```python
from build123d import *

# Parameters (mm, degrees)
CROQUIS1_W              = 56.2
CROQUIS1_H              = 31.2
SALIENTE_EXTRUIR1_DEPTH = 6
CROQUIS3_W              = 51.9
CROQUIS3_H              = 26.9
CORTAR_EXTRUIR1_DEPTH   = 3
CROQUIS5_W              = 56.2
CROQUIS5_H              = 18
SALIENTE_EXTRUIR2_DEPTH = 8
CROQUIS6_W              = 13.3
CROQUIS6_H              = 3.9
CORTAR_EXTRUIR2_DEPTH   = 64.385171768
CROQUIS7_W              = 13.1
CROQUIS7_H              = 8
CORTAR_EXTRUIR3_DEPTH   = 57.729533754
REDONDEO3_R             = 3


with BuildPart() as part:
    # Croquis1 → Saliente-Extruir1 (new body)
    with BuildSketch(Plane(origin=(0, 0, 0), x_dir=(1, 0, 0), z_dir=(0, 1, 0))):
        with Locations((25.1, 12.6)):
            Rectangle(CROQUIS1_W, CROQUIS1_H)
    extrude(amount=SALIENTE_EXTRUIR1_DEPTH)

    # Croquis3 → Cortar-Extruir1 (cut)
    with BuildSketch(Plane(origin=(0, 6, 0), x_dir=(1, 0, 0), z_dir=(0, 1, 0))):
        with Locations((25.1, 12.6)):
            Rectangle(CROQUIS3_W, CROQUIS3_H)
    extrude(amount=-CORTAR_EXTRUIR1_DEPTH, mode=Mode.SUBTRACT)

    # Croquis5 → Saliente-Extruir2 (add)
    with BuildSketch(Plane.XZ):
        with Locations((25.1, -6)):
            Rectangle(CROQUIS5_W, CROQUIS5_H)
    extrude(amount=SALIENTE_EXTRUIR2_DEPTH)

    # Croquis6 → Cortar-Extruir2 (cut, through all)
    with BuildSketch(Plane.ZY.offset(3)):
        with Locations((-8.35, -1.95)):
            Rectangle(CROQUIS6_W, CROQUIS6_H)
    extrude(amount=-CORTAR_EXTRUIR2_DEPTH, mode=Mode.SUBTRACT)

    # Croquis7 → Cortar-Extruir3 (cut, through all)
    with BuildSketch(Plane(origin=(0, 0, -15), x_dir=(-1, 0, 0), z_dir=(0, 0, -1))):
        with Locations((-46.65, -4)):
            Rectangle(CROQUIS7_W, CROQUIS7_H)
        with Locations((-3.55, -4)):
            Rectangle(CROQUIS7_W, CROQUIS7_H)
    extrude(amount=-CORTAR_EXTRUIR3_DEPTH, mode=Mode.SUBTRACT)

    # Redondeo3
    redondeo3_edges = [part.edges().sort_by_distance(p)[0] for p in [
        (-3, 3, -28.2),
        (53.2, 3, -28.2),
        (53.2, 3, 3),
        (-3, 3, 3),
    ]]
    fillet(redondeo3_edges, radius=REDONDEO3_R)


solid = part.part
```
Check sheet for the modelled part. Datum: model origin and axes. Units: mm. A direction names the side the tool comes from. Round coordinates to 2 decimals unless told otherwise and drop trailing zeros. Loops run counter-clockwise (first coordinate to the right, second up) from the corner with the lowest first, then second, coordinate; pieces in that order, holes last. Notation, with made-up numbers: M -19,-9.75 L 2,-9.75 A11 ccw 2,6.25 Z; hole C 10,2.25 d11. An arc over 180 degrees is marked long. Answer as a JSON object with one key per item and string values.
1. Scan lines: line 1 (X direction, y = 4.25, z = -13); line 2 (Z direction, x = 46, y = 4); line 3 (Y direction, x = 27, z = -17.5). Record each from-to range of solid material in increasing order.
Reply:
{"line 1": "x = -3 to -0.85, 51.05 to 53.2", "line 2": "z = -28.2 to -26.05, 0.85 to 3", "line 3": "y = 0 to 3"}
2. Access from +Z, -Z, +X, -X, +Y, -Y to the whole of each face (thin tool, end or side, straight path). Record for faces 5 (the flat face through (51.05, 5, -12)), 6 (the flat face through (25, -3.9, -8)), 7 (the flat face through (25, -6, -15)), 8 (the flat face through (10.1, -5, -4)), 9 (the flat face through (-3, 3, -13)).
Reply:
{"face 5": "+Y", "face 6": "-Z, +X, -X", "face 7": "-Z, +X, -X, -Y", "face 8": "+Z, -Z, -X, -Y", "face 9": "+Z, -Z, -X, +Y, -Y"}
3. Section check D-D (y = -7). Record the boundary of the cut face in (x, z).
Reply:
{"outline": "M 10.1,-15 L 40.1,-15 L 40.1,3 L 10.1,3 Z"}
4. Section check C-C (z = -17.5). Record the boundary of the cut face in (x, y).
Reply:
{"outline": "M -3,0 L 53.2,0 L 53.2,6 L 51.05,6 L 51.05,3 L -0.85,3 L -0.85,6 L -3,6 Z"}
5. Section check A-A (z = -11.5). Record the boundary of the cut face in (x, y), plus the area to 4 significant figures.
Reply:
{"outline": "M -3,0 L 53.2,0 L 53.2,6 L 51.05,6 L 51.05,3 L -0.85,3 L -0.85,6 L -3,6 Z; M 10.1,-8 L 40.1,-8 L 40.1,-3.9 L 10.1,-3.9 Z", "area": "304.5 mm²"}
6. Mould release check, pull along Y, two halves, no side actions. Record for faces 1 (the flat face through (25, 1, 3)), 2 (the flat face through (25, -2, -1.7)), 3 (the flat face through (25, 3, -13)), 4 (the flat face through (25, -8, -6)): pulls with the +Y half, pulls with the -Y half, needs draft (parallel to the pull), parting line crosses it, or undercut.
Reply:
{"face 1": "needs draft", "face 2": "undercut", "face 3": "pulls with the +Y half", "face 4": "pulls with the -Y half"}
7. Gauge pin test, flat ends, axial feed: P1, Ø2, axis at x = 23, y = -6.5, coming from the -Z side; P2, Ø5, axis at x = 18.5, z = -18.5, coming from the +Y side; P3, Ø15.5, axis at x = 15, z = -16, coming from the -Y side; P4, Ø6, axis at x = 6, z = -4, coming from the -Y side. Record the tip position at first contact, or that the pin passes through.
Reply:
{"P1": "stops at z = -15", "P2": "stops at y = 3", "P3": "stops at y = -8", "P4": "stops at y = 0"}
8. Section check B-B (x = 21.5). Record the boundary of the cut face in (y, z).
Reply:
{"outline": "M -8,-15 L -3.9,-15 L -3.9,-1.7 L 0,-1.7 L 0,-28.2 L 6,-28.2 L 6,-26.05 L 3,-26.05 L 3,0.85 L 6,0.85 L 6,3 L -8,3 Z"}
